For this review, take the finished solid that the model builds, in its own axes (mm). Face numbers are marked on the shaded views. A direction names the side the tool comes from. Round coordinates to 2 decimals unless told otherwise and drop trailing zeros. Write each loop counter-clockwise with the first axis right and the second up, starting at its lowest first coordinate (ties: lowest second). Pieces come first, ordered by that corner, then holes. Notation, with made-up numbers: (65.25, 26) - (96.25, 26) arc R16 ccw to (96.25, 50) - close; hole circle Ø6 at (38, -25). An arc over 180 degrees is marked (long way). One line per item, written item: value. Start each with the question number.
Q1. Add section B-B on y = 0. Give the number of separate pieces and of enclosed holes in the cut face, and give its area (3 significant figures).
Q2. Add section D-D on y = -8.25. Write out the cut boundary in (x, z), and give its area (3 significant figures).
Q3. Add section C-C on x = 13. Write out the cut boundary in (y, z), and give its area (3 significant figures).
Q4. For probe 1 along X at (y, z) = (7, 13.5); probe 2 along Y at (x, z) = (-18.05, 52); probe 3 along X at (y, z) = (-9, 44), list the stretches that pass through material, from the lowest coordinate up.
Q5. Tool access review of the marked faces 4, 5, 6, 7 and 8: name each direction out of +Z, -Z, +X, -X, +Y, -Y from which nothing blocks a thin tool from reaching the whole face with its end or side.
Q6. Mouldability with a two-part tool opening along Y and no side actions: class the marked faces 1, 2 and 3 as +Y half, -Y half, draft (parallel to the pull), parting line (faces both ways), or undercut.
Q7. Add section A-A on z = 52. Write out the cut boundary in (x, y).
Q8. Clearance check with flat-ended pins moving along their axes: pin 1 Ø8 at (x, y) = (-10, 0) entering from -Z; pin 2 Ø6.5 at (y, z) = (-2, 50.5) entering from +X; pin 3 Ø11.5 at (y, z) = (0, 52) entering from -X. State where each tip first meets the part, or that it passes through.
```python
from build123d import *

# Parameters (mm, degrees)
SKETCH_1_W               = 44
SKETCH_1_H               = 20
EXTRUDE_1_DEPTH          = 70
SKETCH_2_W               = 22
SKETCH_2_H               = 20
CUT_EXTRUDE_1_DEPTH      = 40
SKETCH_3_R               = 4.5
CUT_EXTRUDE_2_DEPTH      = 50
SKETCH_4_R               = 6.5
CUT_EXTRUDE_4_DEPTH      = 5
SKETCH_5_R               = 3
CUT_EXTRUDE_5_DEPTH      = 29
CUT_EXTRUDE_6_DEPTH      = 5
CUT_EXTRUDE_6_DEPTH_BACK = 5


with BuildPart() as part:
    # Sketch 1 → Extrude 1 (new body)
    with BuildSketch(Plane.XY):
        Rectangle(SKETCH_1_W, SKETCH_1_H)
    extrude(amount=EXTRUDE_1_DEPTH)

    # Sketch 2 → Cut-Extrude 1 (cut)
    with BuildSketch(Plane.XY.offset(70)):
        with Locations((-0.092136373, 0)):
            Rectangle(SKETCH_2_W, SKETCH_2_H)
    extrude(amount=-CUT_EXTRUDE_1_DEPTH, mode=Mode.SUBTRACT)

    # Sketch 3 → Cut-Extrude 2 (cut)
    with BuildSketch(Plane(origin=(22, 0, 0), x_dir=(0, 0, -1), z_dir=(1, 0, 0))):
        with Locations((-52, 0)):
            Circle(SKETCH_3_R)
    extrude(amount=-CUT_EXTRUDE_2_DEPTH, mode=Mode.SUBTRACT)

    # Sketch 4 → Cut-Extrude 4 (cut)
    with BuildSketch(Plane.ZY.offset(-22)):
        with Locations((52, 0)):
            Circle(SKETCH_4_R)
    cut_extrude_4 = extrude(amount=CUT_EXTRUDE_4_DEPTH, mode=Mode.SUBTRACT)

    # Sketch 5 → Cut-Extrude 5 (cut)
    with BuildSketch(Plane(origin=(0, 10, 0), x_dir=(1, 0, 0), z_dir=(0, 1, 0))):
        with Locations(Location((13, -13.5, 0), (0, 0, 270))):
            Circle(SKETCH_5_R)
    cut_extrude_5 = extrude(amount=-CUT_EXTRUDE_5_DEPTH, mode=Mode.SUBTRACT)

    # Mirror 2: Cut-Extrude 4, Cut-Extrude 5 across plane
    add(cut_extrude_4.mirror(Plane(origin=(0, 0, 0), x_dir=(0, 0, 1), z_dir=(1, 0, 0))), mode=Mode.SUBTRACT)
    add(cut_extrude_5.mirror(Plane(origin=(0, 0, 0), x_dir=(0, 0, 1), z_dir=(1, 0, 0))), mode=Mode.SUBTRACT)

    # Sketch 6 → Cut-Extrude 6 (cut, two sides: drawn at the far end of the back side and taken through both)
    with BuildSketch(Plane(origin=(0, 0, 0), x_dir=(1, 0, 0), z_dir=(0, 1, 0)).offset(-CUT_EXTRUDE_6_DEPTH_BACK)):
        Polygon((2.5, -24), (2.5, 0), (22, 0), (22, -19.349242405), (17.349242405, -24), align=None)
        Polygon((-22, -19.349242405), (-22, 0), (-2.5, 0), (-2.5, -24), (-17.349242405, -24), align=None)
    extrude(amount=CUT_EXTRUDE_6_DEPTH + CUT_EXTRUDE_6_DEPTH_BACK, mode=Mode.SUBTRACT)


solid = part.part
```
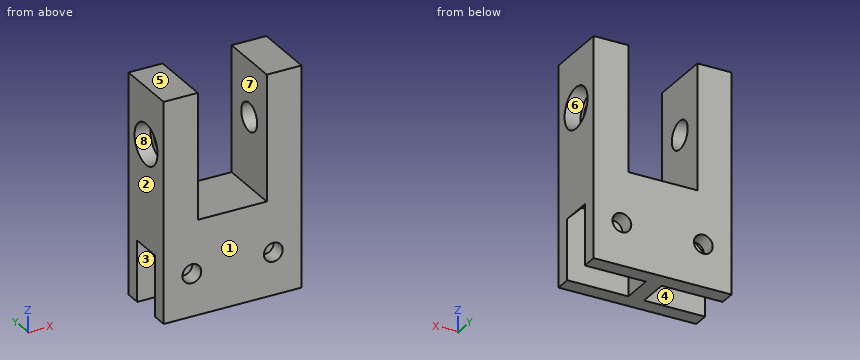
Result set:
1. separate pieces: 3
1. enclosed holes: 0
1. area: 1,050 mm^2
2. outline: (-22, 0) - (22, 0) - (22, 70) - (10.91, 70) - (10.91, 30) - (-11.09, 30) - (-11.09, 70) - (-22, 70) - close; hole circle Ø6 at (-13, 13.5); hole circle Ø6 at (13, 13.5)
2. area: 2,140 mm^2
3. outline: (-10, 0) - (-5, 0) - (-5, 10.5) - (-10, 10.5) - close; (-10, 16.5) - (-5, 16.5) - (-5, 24) - (5, 24) - (5, 16.5) - (10, 16.5) - (10, 70) - (-10, 70) - close; (5, 0) - (10, 0) - (10, 10.5) - (5, 10.5) - close; hole circle Ø9 at (0, 52)
3. area: 1,040 mm^2
4. probe 1: x = -22 to -16, -10 to 10, 16 to 22
4. probe 2: y = -10 to -6.5, 6.5 to 10
4. probe 3: x = -22 to -11.09, 10.91 to 22
5. face 4: -Z
5. face 5: +Z, +X, -X, +Y, -Y
5. face 6: +X
5. face 7: +Z, +Y, -Y
5. face 8: -X
6. face 1: -Y half
6. face 2: draft
6. face 3: undercut
7. outline: (-22, -10) - (-11.09, -10) - (-11.09, -4.5) - (-17, -4.5) - (-17, -6.5) - (-22, -6.5) - close; (-22, 6.5) - (-17, 6.5) - (-17, 4.5) - (-11.09, 4.5) - (-11.09, 10) - (-22, 10) - close; (10.91, -10) - (22, -10) - (22, -6.5) - (17, -6.5) - (17, -4.5) - (10.91, -4.5) - close; (10.91, 4.5) - (17, 4.5) - (17, 6.5) - (22, 6.5) - (22, 10) - (10.91, 10) - close
8. pin 1: stops at z = 24
8. pin 2: stops at x = 17
8. pin 3: stops at x = -17
